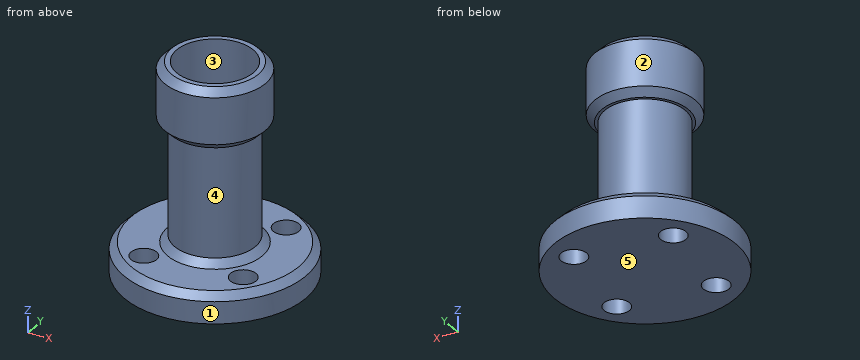
Autodesk Inventor part; units mm, degrees
ref_plane "YZ Plane" through (0, 0, 0) normal (1, 0, 0) x (0, 1, 0)
ref_plane "XZ Plane" through (0, 0, 0) normal (0, 1, 0) x (-1, 0, 0)
ref_plane "XY Plane" through (0, 0, 0) normal (0, 0, 1) x (1, 0, 0)
sketch "Sketch1" plane through (0, 0, 0) normal (0, 0, 1) x (1, 0, 0)
  line L0 (-438.4859, 117.5453) -> (-265.3275, 117.5453) construction
  line L1 (-265.3275, 117.5453) -> (-265.3275, -22.5902) construction
  line L2 (-265.3275, -22.5902) -> (-438.4859, -22.5902) construction
  line L3 (-438.4859, -22.5902) -> (-438.4859, 117.5453) construction
  circle A0 centre (0, 0) radius 45
  dimension "d3" = 90
extrude "Extrusion1" add sketch "Sketch1" along normal blind 8 and the other way blind 6.4
sketch "Sketch2" plane through (0, 0, 8) normal (0, 0, 1) x (1, 0, 0)
  circle A0 centre (19.5689, 25.9482) radius 6.35
  circle A1 centre (-25.9482, 19.5689) radius 6.35
  circle A2 centre (-19.5689, -25.9482) radius 6.35
  circle A3 centre (25.9482, -19.5689) radius 6.35
  point P0 (0, 0)
  dimension "d7" = 12.7
  dimension "d8" = 32.5
  dimension "d11" = 360
extrude "Extrusion2" cut sketch "Sketch2" against normal through all
sketch "Sketch3" plane through (0, 0, 8) normal (0, 0, 1) x (1, 0, 0)
  circle A0 centre (0, 0) radius 20
  circle A1 centre (0, 0) radius 15
  dimension "d16" = 40
  dimension "d17" = 30
extrude "Extrusion3" add sketch "Sketch3" along normal blind 64.4
sketch "Sketch4" plane through (0, 0, 72.4) normal (0, 0, 1) x (1, 0, 0)
  circle A0 centre (0, 0) radius 25
  circle A1 centre (0, 0) radius 15
  circle A2 centre (0, 0) radius 19
  dimension "d20" = 50
  dimension "d21" = 38
extrude "Extrusion4" add sketch "Sketch4" along normal blind 24 and the other way blind 6 contours A0
chamfer "Chamfer1" distance 3.5 angle 45 1 edges at (-20, 0, 8)
chamfer "Chamfer2" distance 3.5 angle 45 1 edges at (-25, 0, 96.4)
chamfer "Chamfer3" distance 3.5 angle 45 1 edges at (-25, 0, 66.4)
chamfer "Chamfer4" distance 3.5 angle 45 1 edges at (-45, 0, 8)
properties part number "cad@23"
Read the model definition and answer for the solid it produces. Units are mm, in the model's axes. Face numbers are marked on the shaded views. A direction names the side the tool comes from. Coordinates: 2 decimals unless noted, no trailing zeros. Loops run counter-clockwise (first coordinate to the right, second up) from the corner with the lowest first, then second, coordinate; pieces in that order, holes last. Notation, with made-up numbers: (-18, 53.5) -> (-3, 53.5) arc R29 cw to (-3, 83.5) -> close; hole circle Ø2 at (12.5, 7.25). An arc over 180 degrees is marked (long way). Write item = value, one per line. Start each with the question number.
1) The part is cut by section A-A, the plane y = 0. Determine the outline of the cut face in (x, z), plus the area to 3 significant figures.
2) The part is cut by section C-C, the plane z = 13.5. Determine the outline of the cut face in (x, y), plus the area to 3 significant figures.
3) For the marked faces 1 and 2, determine the directions among +Z, -Z, +X, -X, +Y, -Y from which every point of the face is accessible in a straight line to the end or side of a thin tool.
4) Find the intervals of material crossed by L1, parallel to Y at x = 0, z = 41; L2, parallel to Z at x = -34, y = -12.5; L3, parallel to Y at x = -1.5, z = 42, in increasing order. Write a range as from..to.
5) Given P1, Ø16.5, axis at x = 25.95, y = -19.57, coming from the -Z side; P2, Ø1.5, axis at y = 0.5, z = 40, coming from the -X side; P3, Ø1.5, axis at y = -32, z = 4, coming from the -X side; P4, Ø2, axis at x = 16.5, z = 35, coming from the -Y side, each flat-ended and moving along its own axis, determine where each tip first touches the part or whether it passes through.
6) The mould has two halves that part along X. Classify the marked faces 3, 4 and 5: pulls with the +X half, pulls with the -X half, needs draft (parallel to the pull), parting line crosses it, or undercut.
Result:
q1.outline = (-45, -6.4) -> (45, -6.4) -> (45, 4.5) -> (41.5, 8) -> (23.5, 8) -> (20, 11.5) -> (20, 66.4) -> (21.5, 66.4) -> (25, 69.9) -> (25, 92.9) -> (21.5, 96.4) -> (19, 96.4) -> (19, 72.4) -> (15, 72.4) -> (15, 8) -> (-15, 8) -> (-15, 72.4) -> (-19, 72.4) -> (-19, 96.4) -> (-21.5, 96.4) -> (-25, 92.9) -> (-25, 69.9) -> (-21.5, 66.4) -> (-20, 66.4) -> (-20, 11.5) -> (-23.5, 8) -> (-41.5, 8) -> (-45, 4.5) -> close
q1.area = 2,260 mm²
q2.outline = circle Ø40 at (0, 0); hole circle Ø30 at (0, 0)
q2.area = 550 mm²
q3.face_1 = +Z, -Z
q3.face_2 = +Z
q4.L1 = -20..-15, 15..20
q4.L2 = -6.4..8
q4.L3 = -19.94..-14.92, 14.92..19.94
q5.P1 = -6.4
q5.P2 = -20
q5.P3 = -32.38
q5.P4 = -12.64
q6.face_3 = undercut
q6.face_4 = parting line crosses it
q6.face_5 = needs draft
